from build123d import *

# Parameters (mm, degrees)
ESQUISSE1_W             = 20
ESQUISSE1_H             = 148.25
ESQUISSE2_R             = 55
ENL_V_MAT_EXTRU_1_DEPTH = 211.608938557
ESQUISSE3_R             = 87.63760146
ENL_V_MAT_EXTRU_2_DEPTH = 13
TROU_TARAUD_M101_D      = 8.5


with BuildPart() as part:
    # Esquisse1 → Révolution1 (revolve)
    with BuildSketch(Plane.XY, mode=Mode.PRIVATE) as r_volution1_sk:
        with Locations((397.851746626, 74.125)):
            Rectangle(ESQUISSE1_W, ESQUISSE1_H)
    revolve(r_volution1_sk.sketch.rotate(Axis((22.672384616, 0, 0), (1, 0, 0)), 90), axis=Axis((22.672384616, 0, 0), (1, 0, 0)))

    # Esquisse2 → Enlèv. mat.-Extru.1 (cut, through all)
    with BuildSketch(Plane(origin=(407.851746626, 0, 0), x_dir=(0, 0, -1), z_dir=(1, 0, 0))):
        Circle(ESQUISSE2_R)
    extrude(amount=-ENL_V_MAT_EXTRU_1_DEPTH, mode=Mode.SUBTRACT)

    # Esquisse3 → Enlèv. mat.-Extru.2 (cut)
    with BuildSketch(Plane.ZY.offset(-387.851746626)):
        Circle(ESQUISSE3_R)
    extrude(amount=-ENL_V_MAT_EXTRU_2_DEPTH, mode=Mode.SUBTRACT)

    # Trou taraudé M101 (through all)
    with Locations(Plane(origin=(387.851746626, 130, 0), x_dir=(0, 0, -1), z_dir=(-1, 0, 0))):
        with Locations((0, 0), (130, 130), (0, 260), (-130, 130)):
            Hole(TROU_TARAUD_M101_D / 2)


solid = part.part
Could you check a few things on this model? Use its own coordinates, in mm. A direction names the side the tool comes from. Give positions to 0.01 mm unless a question says otherwise; leave off trailing zeros. Order: outer loops, then holes, each group sorted by start corner. A loop starts at its lowest first (then second) coordinate and runs counter-clockwise, first axis right, second up.
Item 1: If we mould it in two halves opening along Z, with no side actions, what happens to faces 1 (the face through (397.992, -125.005, 79.698)), 2 (the face through (407.852, -2, -64)), 3 (the face through (397.992, -134.214, -0.553))? For each: pulls with the +Z half, pulls with the -Z half, needs draft (parallel to the pull), parting line crosses it, or undercut.
Item 2: For faces 4 (the face through (400.852, 40, 38)), 5 (the face through (397.992, 125.786, -0.553)), which set-ups out of +Z, -Z, +X, -X, +Y, -Y let a thin tool reach every point of the face, with its end or its side?
Item 3: If we section it at C-C, the plane x = 397.25: Write out the boundary of the cut face in (y, z).
Item 4: I'm going to push flat-ended pins straight in: pin 1 (6 mm diameter, centred on x = 403, z = -76.5, fed in from -Y); pin 2 (2 mm diameter, centred on x = 399, y = 16.5, fed in from -Z); pin 3 (1 mm diameter, centred on x = 402, z = -116, fed in from -Y); pin 4 (5 mm diameter, centred on y = 0, z = 130, fed in from -X). Where does each tip first touch, or does it pass through?
Item 5: I need wall thicknesses on line 1 (Y direction, x = 398, z = -0.5); line 2 (Z direction, x = 396, y = -130); line 3 (Z direction, x = 392.75, y = -53). Which ranges of each line are inside material? Lowest first, please.
Item 6: If we section it at B-B, the plane y = -44.5: Write out the boundary of the cut face in (x, z), plus the area to 3 significant figures.
Item 7: If we section it at A-A, the plane z = -49: Write out the boundary of the cut face in (x, y), plus the area to 3 significant figures.
Item 8: If we section it at D-D, the plane y = 0: Write out the boundary of the cut face in (x, z).
Values:
1. face 1: parting line crosses it
1. face 2: needs draft
1. face 3: undercut
2. face 4: -X
2. face 5: +X, -X
3. outline: circle Ø296.5 at (0, 0); hole circle Ø8.5 at (-130, 0); hole circle Ø175.28 at (0, 0); hole circle Ø8.5 at (0, -130); hole circle Ø8.5 at (0, 130); hole circle Ø8.5 at (130, 0)
4. pin 1: stops at y = -128.75
4. pin 2: stops at z = -147.44
4. pin 3: stops at y = -92.94
4. pin 4: passes through
5. line 1: y = -148.25 to -134.22, -125.78 to -87.64, 87.64 to 125.78, 134.22 to 148.25
5. line 2: z = -71.26 to -4.25, 4.25 to 71.26
5. line 3: z = -138.45 to -69.8, 69.8 to 138.45
6. outline: (387.85, -141.41) - (407.85, -141.41) - (407.85, -32.32) - (400.85, -32.32) - (400.85, -75.5) - (387.85, -75.5) - close; (387.85, 75.5) - (400.85, 75.5) - (400.85, 32.32) - (407.85, 32.32) - (407.85, 141.41) - (387.85, 141.41) - close
6. area: 3,240 mm2
7. outline: (387.85, -139.92) - (407.85, -139.92) - (407.85, -24.98) - (400.85, -24.98) - (400.85, -72.66) - (387.85, -72.66) - close; (387.85, 72.66) - (400.85, 72.66) - (400.85, 24.98) - (407.85, 24.98) - (407.85, 139.92) - (387.85, 139.92) - close
7. area: 3,360 mm2
8. outline: (387.85, -148.25) - (407.85, -148.25) - (407.85, -134.25) - (387.85, -134.25) - close; (387.85, -125.75) - (407.85, -125.75) - (407.85, -55) - (400.85, -55) - (400.85, -87.64) - (387.85, -87.64) - close; (387.85, 87.64) - (400.85, 87.64) - (400.85, 55) - (407.85, 55) - (407.85, 125.75) - (387.85, 125.75) - close; (387.85, 134.25) - (407.85, 134.25) - (407.85, 148.25) - (387.85, 148.25) - close
